from build123d import *

# Parameters (mm, degrees)
F1_DEPTH = 8


with BuildPart() as f1:
    # F0 (on Top) → F1 (new body)
    with BuildSketch(Plane.XY):
        Polygon((-8.791217, 10.820824), (-8.791217, 15.58735), (-1.791217, 15.58735), (-1.791217, 0), (0, 0), (2.168675, 0), (2.168675, 7.725904), (4.33735, 7.725904), (4.33735, 13.147592), (6.77711, 13.147592), (9.759036, 15.58735), (11.755203, 13.147592), (11.755203, 7.725904), (17.3494, 7.725904), (17.3494, 30.496988), (26.024099, 30.496988), (26.024099, 7.725904), (26.024099, 0), (30.903617, 0), (30.903617, 19.495524), (30.903617, 24.262048), (33.421363, 27.499158), (34.764209, 26.454724), (36.612159, 26.454724), (36.612159, 24.262048), (36.612159, 0), (40.858796, 0), (40.858796, 19.495524), (44.108796, 25.124689), (47.358796, 19.495524), (47.358796, 8.10998), (50.963856, 8.10998), (50.963856, 3.388554), (54.483884, 3.388554), (54.483884, 26.713658), (58.685689, 33.991398), (62.887494, 26.713658), (62.887494, 3.388554), (67.212614, 3.388554), (67.212614, 8.810241), (71.00779, 8.810241), (71.00779, 3.388554), (74.802975, 3.388554), (74.802975, 0), (75.802975, 0), (75.802975, 4.388554), (74.802975, 4.388554), (72.00779, 4.388554), (72.00779, 9.810241), (68.572836, 9.810241), (66.212614, 9.810241), (66.212614, 6.689354), (66.212614, 4.388554), (64.699309, 4.388554), (63.875258, 4.388554), (63.887494, 26.713658), (58.694566, 35.708074), (53.483884, 26.682909), (53.483884, 4.388554), (51.963856, 4.388554), (51.963856, 9.10998), (48.358796, 9.10998), (48.358796, 19.495524), (44.108796, 26.85674), (39.858796, 19.495524), (39.858796, 1), (37.612159, 1), (37.612159, 27.454724), (34.764209, 27.454724), (34.232993, 27.867891), (33.421363, 28.499158), (29.903617, 24.262048), (29.903617, 1), (27.024099, 1), (27.024099, 31.496988), (16.3494, 31.496988), (16.3494, 8.725904), (12.755203, 8.725904), (12.755203, 13.147592), (9.759036, 16.58735), (6.77711, 14.147592), (4.33735, 14.147592), (3.33735, 14.147592), (3.33735, 8.725904), (1.168675, 8.725904), (1.168675, 1), (-0.791217, 1), (-0.791217, 16.58735), (-9.791217, 16.58735), (-9.791217, 11.820824), (-16.291217, 11.820824), (-16.291217, 1), (-21.771085, 1), (-21.771085, 11.820824), (-25.821578, 11.820824), (-25.821578, 20.495524), (-30.47494, 20.495524), (-36.512049, 20.495524), (-36.512049, 1), (-40.204821, 1), (-40.204821, 24.262048), (-44.357452, 31.454616), (-48.510083, 24.262048), (-48.510083, 1), (-55.096389, 1), (-55.096389, 14.208821), (-61.347563, 14.208821), (-61.347563, 16.556969), (-66.283464, 16.556969), (-66.144578, 0), (-65.144543, 0), (-65.275041, 15.556969), (-62.351945, 15.581489), (-62.347563, 15.059114), (-62.347563, 13.208821), (-56.096389, 13.208821), (-56.096389, 0), (-51.847431, 0), (-47.510083, 0), (-47.510083, 24.262048), (-44.357452, 29.722565), (-41.204821, 24.262048), (-41.204821, 0), (-35.512049, 0), (-35.512049, 19.495524), (-26.821578, 19.495524), (-26.821578, 10.820824), (-22.771085, 10.820824), (-22.771085, 0), (-17.891567, 0), (-15.291217, 0), (-15.291217, 1), (-15.291217, 10.820824), align=None)
        Polygon((0, 0), (-1.791217, 0), (-15.291217, 0), (-17.891567, 0), (-22.771085, 0), (-35.512049, 0), (-41.204821, 0), (-47.510083, 0), (-51.847431, 0), (-56.096389, 0), (-65.144543, 0), (-66.144578, 0), (-71.747227, -0.046997), (-71.730845, -2), (74.802975, -2), (75.802975, -2), (75.802975, 0), (74.802975, 0), (40.858796, 0), (36.612159, 0), (30.903617, 0), (26.024099, 0), (2.168675, 0), align=None)
    extrude(amount=F1_DEPTH)


solid = f1.part
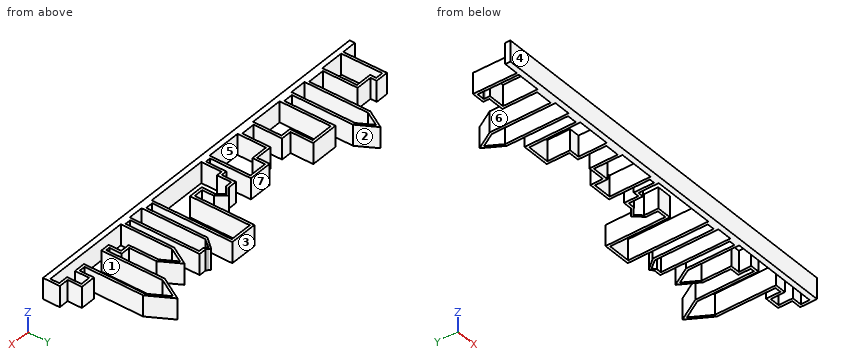
Design review of the part built by this model. Coordinates are the model's own, in mm. Face numbers are marked on the shaded views. A direction names the side the tool comes from. Coordinates: 2 decimals unless noted, no trailing zeros. Order: outer loops, then holes, each group sorted by start corner. A loop starts at its lowest first (then second) coordinate and runs counter-clockwise, first axis right, second up.
Item 1: For line 1 (Y direction, x = 25.5, z = 3); line 2 (Y direction, x = 65, z = 7.5); line 3 (Y direction, x = 2, z = 7.75), list the stretches that pass through material, from the lowest coordinate up.
Item 2: The part is to be moulded in two halves that separate along Y. For the marked faces 4, 5, 6 and 7, say which applies: pulls with the +Y half, pulls with the -Y half, needs draft (parallel to the pull), parting line crosses it, or undercut.
Item 3: For the marked faces 1, 2 and 3, list the 3-axis set-ups (+Z, -Z, +X, -X, +Y, -Y) from which the entire face can be reached by the end or side of a thin tool; tool diameter is ignored.
Item 4: For pin 1 Ø1.5 at (y, z) = (23.5, 5.5) entering from +X; pin 2 Ø2 at (x, y) = (6, 16) entering from -Z; pin 3 Ø3.5 at (y, z) = (10.5, 2.5) entering from +X; pin 4 Ø3 at (x, z) = (-39, 4.5) entering from +Y, all flat-tipped, find the tip position at first contact; note any pin that passes through.
Item 5: Take a section at A-A, the plane z = 3.5. Count the separate pieces of the cut face and the enclosed holes in it, then the cut area to 3 significant figures.
Item 6: Take a section at C-C, the plane x = -51. Write out the cut boundary in (y, z), then the cut area to 3 significant figures.
The answers:
1. line 1: y = -2 to 0, 30.5 to 31.5
1. line 2: y = -2 to 0, 3.39 to 4.39
1. line 3: y = -2 to 8.73
2. face 4: pulls with the -Y half
2. face 5: undercut
2. face 6: needs draft
2. face 7: pulls with the +Y half
3. face 1: +Z, -Z
3. face 2: +Z, -Z, +Y
3. face 3: +Z, -Z, -X, +Y
4. pin 1: stops at x = 63.89
4. pin 2: passes through
4. pin 3: stops at x = 72.01
4. pin 4: stops at y = 24.77
5. separate pieces: 1
5. enclosed holes: 7
5. area: 820 mm2
6. outline: (-2, 0) - (1, 0) - (1, 8) - (-2, 8) - close
6. area: 24.0 mm2
